```python
from build123d import *

# Parameters (mm, degrees)
SKETCH1_W           = 24.274152736
SKETCH1_H           = 45.799920806
SKETCH1_R           = 4.25
BOSS_EXTRUDE1_DEPTH = 2
SKETCH1_3_W         = 24.274152736
SKETCH1_3_H         = 2
SKETCH1_3_H_2       = 43.799920806
BOSS_EXTRUDE2_DEPTH = 8
BOSS_EXTRUDE3_START = -8
SKETCH1_4_W         = 24.274152736
SKETCH1_4_H         = 43.799920806
SKETCH1_4_W_2       = 10
SKETCH1_4_H_2       = 11
SKETCH1_4_H_3       = 2
SKETCH1_4_W_3       = 14.274152736
SKETCH1_4_R         = 1.5
SKETCH1_4_W_4       = 10.725847264
BOSS_EXTRUDE3_DEPTH = 3
SKETCH1_5_R         = 4.25
BOSS_EXTRUDE4_DEPTH = 11
SKETCH2_R           = 4.25
SKETCH2_R_2         = 1.5
CUT_EXTRUDE1_DEPTH  = 3
SKETCH2_2_R         = 1.5
CUT_EXTRUDE2_DEPTH  = 14


with BuildPart() as part:
    # Sketch1 → Boss-Extrude1 (new body)
    with BuildSketch(Plane.XY):
        with Locations((-69.637076368, 28.899960403)):
            Rectangle(SKETCH1_W, SKETCH1_H)
        with Locations((-68.922189075, 39.999920806)):
            Circle(SKETCH1_R, mode=Mode.SUBTRACT)
    extrude(amount=BOSS_EXTRUDE1_DEPTH)

    # Sketch1<3> → Boss-Extrude2 (add)
    with BuildSketch(Plane.XY):
        with Locations((-69.637076368, 7)):
            Rectangle(SKETCH1_3_W, SKETCH1_3_H)
        with Locations((-69.637076368, 29.899960403)):
            Rectangle(SKETCH1_3_W, SKETCH1_3_H_2)
        Polygon((-61.070225414, 39.999920806), (-64.996207244, 33.199920806), (-72.848170905, 33.199920806), (-76.774152736, 39.999920806), (-72.848170905, 46.799920806), (-64.996207244, 46.799920806), align=None, mode=Mode.SUBTRACT)
    extrude(amount=-BOSS_EXTRUDE2_DEPTH)

    # Sketch1<4> → Boss-Extrude3 (add)
    with BuildSketch(Plane.XY.offset(BOSS_EXTRUDE3_START)):
        with Locations((-69.637076368, 29.899960403)):
            Rectangle(SKETCH1_4_W, SKETCH1_4_H)
        Polygon((-61.070225414, 39.999920806), (-64.996207244, 33.199920806), (-72.848170905, 33.199920806), (-76.774152736, 39.999920806), (-72.848170905, 46.799920806), (-64.996207244, 46.799920806), align=None, mode=Mode.SUBTRACT)
        with Locations((-62.5, 0)):
            Rectangle(SKETCH1_4_W_2, SKETCH1_4_H_2)
        Polygon((-59.035898385, 0), (-60.767949192, 3), (-64.232050808, 3), (-65.964101615, 0), (-64.232050808, -3), (-60.767949192, -3), align=None, mode=Mode.SUBTRACT)
        Polygon((-67.5, 5.5), (-57.5, 5.5), (-57.5, 6), (-81.774152736, 6), (-81.774152736, 5.5), align=None)
        with Locations((-69.637076368, 7)):
            Rectangle(SKETCH1_4_W, SKETCH1_4_H_3)
        with Locations((-74.637076368, 0)):
            Rectangle(SKETCH1_4_W_3, SKETCH1_4_H_2)
        Polygon((-60.767949192, -3), (-59.035898385, 0), (-60.767949192, 3), (-64.232050808, 3), (-65.964101615, 0), (-64.232050808, -3), align=None)
        with Locations((-62.5, 0)):
            Circle(SKETCH1_4_R, mode=Mode.SUBTRACT)
        with Locations((-87.137076368, 0)):
            Rectangle(SKETCH1_4_W_4, SKETCH1_4_H_2)
        Polygon((-90.5, -1.732050808), (-87.5, -3.464101615), (-84.5, -1.732050808), (-84.5, 1.732050808), (-87.5, 3.464101615), (-90.5, 1.732050808), align=None, mode=Mode.SUBTRACT)
        Polygon((-90.5, 1.732050808), (-90.5, -1.732050808), (-87.5, -3.464101615), (-84.5, -1.732050808), (-84.5, 1.732050808), (-87.5, 3.464101615), align=None)
        with Locations((-87.5, 0)):
            Circle(SKETCH1_4_R, mode=Mode.SUBTRACT)
    extrude(amount=-BOSS_EXTRUDE3_DEPTH)

    # Sketch1<5> → Boss-Extrude4 (add)
    with BuildSketch(Plane.XY):
        Polygon((-76.774152736, 39.999920806), (-72.848170905, 33.199920806), (-64.996207244, 33.199920806), (-61.070225414, 39.999920806), (-64.996207244, 46.799920806), (-72.848170905, 46.799920806), align=None)
        with Locations((-68.922189075, 39.999920806)):
            Circle(SKETCH1_5_R, mode=Mode.SUBTRACT)
    extrude(amount=-BOSS_EXTRUDE4_DEPTH)

    # Sketch2 → Cut-Extrude1 (cut)
    with BuildSketch(Plane.XY.offset(2)):
        with Locations((-68.922189075, 39.999920806)):
            Circle(SKETCH2_R)
        Polygon((-73.45808746, 39.999920806), (-75.190138267, 42.999920806), (-78.654239882, 42.999920806), (-80.38629069, 39.999920806), (-78.654239882, 36.999920806), (-75.190138267, 36.999920806), align=None)
        with Locations((-76.922189075, 39.999920806)):
            Circle(SKETCH2_R_2, mode=Mode.SUBTRACT)
        Polygon((-68.922189075, 28.535819191), (-65.922189075, 30.267869999), (-65.922189075, 33.731971614), (-68.922189075, 35.464022422), (-71.922189075, 33.731971614), (-71.922189075, 30.267869999), align=None)
        with Locations((-68.922189075, 31.999920806)):
            Circle(SKETCH2_R_2, mode=Mode.SUBTRACT)
        Polygon((-68.922189075, 44.535819191), (-65.922189075, 46.267869999), (-65.922189075, 49.731971614), (-68.922189075, 51.464022422), (-71.922189075, 49.731971614), (-71.922189075, 46.267869999), align=None)
        with Locations((-68.922189075, 47.999920806)):
            Circle(SKETCH2_R_2, mode=Mode.SUBTRACT)
        Polygon((-64.38629069, 39.999920806), (-62.654239882, 36.999920806), (-59.190138267, 36.999920806), (-57.45808746, 39.999920806), (-59.190138267, 42.999920806), (-62.654239882, 42.999920806), align=None)
        with Locations((-60.922189075, 39.999920806)):
            Circle(SKETCH2_R_2, mode=Mode.SUBTRACT)
    extrude(amount=-CUT_EXTRUDE1_DEPTH, mode=Mode.SUBTRACT)

    # Sketch2<2> → Cut-Extrude2 (cut, through all)
    with BuildSketch(Plane.XY.offset(2)):
        with Locations((-60.922189075, 39.999920806)):
            Circle(SKETCH2_2_R)
        with Locations((-68.922189075, 47.999920806)):
            Circle(SKETCH2_2_R)
        with Locations((-76.922189075, 39.999920806)):
            Circle(SKETCH2_2_R)
        with Locations((-68.922189075, 31.999920806)):
            Circle(SKETCH2_2_R)
    extrude(amount=-CUT_EXTRUDE2_DEPTH, mode=Mode.SUBTRACT)


solid = part.part
```
Build history of the part. All positions in model axes, mm. A direction names the side the tool comes from. Give positions to 0.01 mm unless a question says otherwise; leave off trailing zeros. Loops run counter-clockwise (first coordinate to the right, second up) from the corner with the lowest first, then second, coordinate; pieces in that order, holes last.
1) Probe line 1 along X through (y, z) = (47.5, -0.25); line 2 along Y through (x, z) = (-87.5, -8.8); line 3 along Z through (x, y) = (-86.5, 2.5). List the from-to ranges inside material, lowest first.
Values follow:
line 1: x = -81.77 to -71.92, -65.92 to -57.5
line 2: y = -5.5 to -1.5, 1.5 to 5.5
line 3: z = -11 to -8
2) Two-plate mould, pull along X, no slides. Class faces 1 (the face through (-61, 37, 1)), 2 (the face through (-73, 29, 2)): released by +X, released by -X, zero draft, split by the parting line, or undercut.
Values follow:
face 1: undercut
face 2: zero draft
3) 3-axis set-ups, long thin cutter, end or side, ignore diameter. For faces 3 (the face through (-70.44, 45.41, 0.52)), 4 (the face through (-75, -5.5, -9)): which of +Z, -Z, +X, -X, +Y, -Y reach the whole face in a straight line?
Values follow:
face 3: +Z
face 4: +Z, -Z, +X, -X, -Y
4) Band-saw the part on D-D on z = -3.5. List the corners of the cut face in (x, y), then the cut area to 3 significant figures.
Values follow:
outline: (-81.77, 6) - (-57.5, 6) - (-57.5, 51.8) - (-81.77, 51.8) - close; hole circle Ø3 at (-76.92, 40); hole circle Ø8.5 at (-68.92, 40); hole circle Ø3 at (-68.92, 32); hole circle Ø3 at (-68.92, 48); hole circle Ø3 at (-60.92, 40)
area: 1,030 mm2
5) Band-saw the part on A-A on x = -87.5. List the corners of the cut face in (y, z), then the cut area to 3 significant figures.
Values follow:
outline: (-5.5, -11) - (-1.5, -11) - (-1.5, -8) - (-5.5, -8) - close; (1.5, -11) - (5.5, -11) - (5.5, -8) - (1.5, -8) - close
area: 24.0 mm2
6) Band-saw the part on C-C on z = -0.25. State how many separate pieces and enclosed holes the cut face has, then the cut area to 3 significant figures.
Values follow:
separate pieces: 1
enclosed holes: 4
area: 930 mm2
7) Band-saw the part on B-B on y = 0. List the corners of the cut face in (x, z), then the cut area to 3 significant figures.
Values follow:
outline: (-92.5, -11) - (-89, -11) - (-89, -8) - (-92.5, -8) - close; (-86, -11) - (-64, -11) - (-64, -8) - (-86, -8) - close; (-61, -11) - (-57.5, -11) - (-57.5, -8) - (-61, -8) - close
area: 87.0 mm2
8) Drop flat-ended pins along their axis: P1, Ø1, axis at x = -76.5, z = -4, coming from the -Y side; P2, Ø2.5, axis at x = -62.5, y = 0, coming from the -Z side; P3, Ø4, axis at x = -76.92, y = 40, coming from the +Z side; P4, Ø3.5, axis at x = -88.5, z = -9.5, coming from the +Y side. Give the stop position or say it passes through.
Values follow:
P1: stops at y = 6
P2: passes through
P3: stops at z = -1
P4: stops at y = 5.5
